Part model, mm, in its own coordinate system. Face numbers are marked on the shaded views. A direction names the side the tool comes from. Coordinates: 2 decimals unless noted, no trailing zeros. Write each loop counter-clockwise with the first axis right and the second up, starting at its lowest first coordinate (ties: lowest second). Pieces come first, ordered by that corner, then holes. Notation, with made-up numbers: M 41.25,52.25 L 69.25,52.25 A25 ccw 69.25,86.25 Z; hole C 84.25,-22.75 d10. An arc over 180 degrees is marked long. Use a Markdown table: item, result. Add a question column.
Q1. Wall check: L1, parallel to Z at x = 16.5, y = 18; L2, parallel to X at y = 5.5, z = 0; L3, parallel to Y at x = -3, z = 14. Give the ranges that are in metal, low to high. Write a range as from..to.
Q2. Slice it at A-A on x = -5. Write the cut outline in (y, z), then the cut area to 3 significant figures.
Q3. Pin check, flat tips, straight feed: pin 1 Ø3 at (x, z) = (4.5, 13.5) entering from -Y; pin 2 Ø6.5 at (x, y) = (-15, 19) entering from -Z; pin 3 Ø2.5 at (x, y) = (14.5, 20.5) entering from +Z. Stop position of each tip, or through.
Q4. Slice it at B-B on y = 6. Write the cut outline in (x, z), then the cut area to 3 significant figures.
Q5. Mould opens along Z. For the marked faces 1, 2 and 3 say: released by +Z, released by -Z, zero draft, split by the parting line, or undercut.
Q6. Slice it at C-C on x = 7. Write the cut outline in (y, z).
Q7. Slice it at D-D on z = 17.5. Write the cut outline in (x, y), then the cut area to 3 significant figures.
Q8. Tool access for the marked faces 4, 5 and 6: list every direction of +Z, -Z, +X, -X, +Y, -Y with a clear straight run to the whole face (end or side of a thin tool).
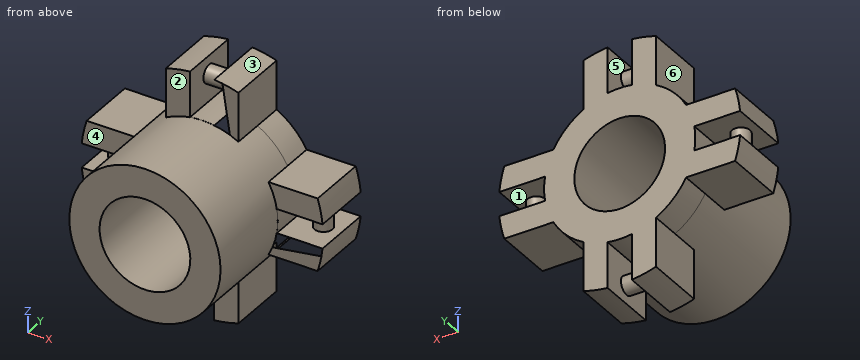
from build123d import *

# Parameters (mm, degrees)
SKETCH1_R           = 12.5
SKETCH1_R_2         = 7.5
BOSS_EXTRUDE1_DEPTH = 20
SKETCH2_R           = 7.5
BOSS_EXTRUDE2_DEPTH = 5
SKETCH3_R           = 1.5
BOSS_EXTRUDE3_DEPTH = 7
CIRPATTERN1_COUNT   = 4


with BuildPart() as part:
    # Sketch1 → Boss-Extrude1 (new body)
    with BuildSketch(Plane(origin=(0, 0, 0), x_dir=(1, 0, 0), z_dir=(0, 1, 0))):
        with Locations(Location((0, 0, 0), (0, 0, 270))):
            Circle(SKETCH1_R)
        with Locations(Location((0, 0, 0), (0, 0, 270))):
            Circle(SKETCH1_R_2, mode=Mode.SUBTRACT)
    extrude(amount=BOSS_EXTRUDE1_DEPTH)

    # Sketch2 → Boss-Extrude2 (add, symmetric)
    with BuildSketch(Plane(origin=(0, 20, 0), x_dir=(1, 0, 0), z_dir=(0, 1, 0))):
        with BuildLine():
            Line((-2, 19.899749), (-2, 12.338963))
            ThreePointArc((-2, 12.338963), (0, 12.5), (2, 12.338963))
            Line((2, 12.338963), (2, 19.899749))
            ThreePointArc((2, 19.899749), (4.021007, 19.591618), (6, 19.078784))
            Line((6, 19.078784), (6, 10.965856))
            ThreePointArc((6, 10.965856), (8.838835, 8.838835), (10.965856, 6))
            Line((10.965856, 6), (19.078784, 6))
            ThreePointArc((19.078784, 6), (19.591618, 4.021007), (19.899749, 2))
            Line((19.899749, 2), (12.338963, 2))
            ThreePointArc((12.338963, 2), (12.5, 0), (12.338963, -2))
            Line((12.338963, -2), (19.899749, -2))
            ThreePointArc((19.899749, -2), (19.591618, -4.021007), (19.078784, -6))
            Line((19.078784, -6), (10.965856, -6))
            ThreePointArc((10.965856, -6), (8.838835, -8.838835), (6, -10.965856))
            Line((6, -10.965856), (6, -19.078784))
            ThreePointArc((6, -19.078784), (4.021007, -19.591618), (2, -19.899749))
            Line((2, -19.899749), (2, -12.338963))
            ThreePointArc((2, -12.338963), (0, -12.5), (-2, -12.338963))
            Line((-2, -12.338963), (-2, -19.899749))
            ThreePointArc((-2, -19.899749), (-4.021007, -19.591618), (-6, -19.078784))
            Line((-6, -19.078784), (-6, -10.965856))
            ThreePointArc((-6, -10.965856), (-8.838835, -8.838835), (-10.965856, -6))
            Line((-10.965856, -6), (-19.078784, -6))
            ThreePointArc((-19.078784, -6), (-19.591618, -4.021007), (-19.899749, -2))
            Line((-19.899749, -2), (-12.338963, -2))
            ThreePointArc((-12.338963, -2), (-12.5, 0), (-12.338963, 2))
            Line((-12.338963, 2), (-19.899749, 2))
            ThreePointArc((-19.899749, 2), (-19.591618, 4.021007), (-19.078784, 6))
            Line((-19.078784, 6), (-10.965856, 6))
            ThreePointArc((-10.965856, 6), (-8.838835, 8.838835), (-6, 10.965856))
            Line((-6, 10.965856), (-6, 19.078784))
            ThreePointArc((-6, 19.078784), (-4.021007, 19.591618), (-2, 19.899749))
        make_face()
        with Locations(Location((0, 0, 0), (0, 0, 270))):
            Circle(SKETCH2_R, mode=Mode.SUBTRACT)
    extrude(amount=BOSS_EXTRUDE2_DEPTH, both=True)

    # Sketch3 → Boss-Extrude3 (add)
    with BuildSketch(Plane.XY.offset(-2)):
        with Locations(Location((-16.899749, 20, 0), (0, 0, 180))):
            Circle(SKETCH3_R)
    boss_extrude3 = extrude(amount=BOSS_EXTRUDE3_DEPTH)

    # CirPattern1: Boss-Extrude3 ×4 about axis
    cirpattern1_axis = Axis((0, 0, 0), (0, -1, 0))
    for i in range(1, CIRPATTERN1_COUNT):
        add(boss_extrude3.rotate(cirpattern1_axis, i * 360 / CIRPATTERN1_COUNT))


solid = part.part
Recorded:
| question | item | result |
|---|---|---|
| 1 | L1 | -6..-2, 2..6 |
| 1 | L2 | -12.5..-7.5, 7.5..12.5 |
| 1 | L3 | 15..25 |
| 2 | outline | M 0,-11.46 L 15,-11.46 L 15,-19.36 L 25,-19.36 L 25,-5.59 L 0,-5.59 Z; M 0,5.59 L 25,5.59 L 25,19.36 L 15,19.36 L 15,11.46 L 0,11.46 Z |
| 2 | area | 451 mm² |
| 3 | pin 1 | y = 15 |
| 3 | pin 2 | z = -6 |
| 3 | pin 3 | z = 6 |
| 4 | outline | C 0,0 d25; hole C 0,0 d15 |
| 4 | area | 314 mm² |
| 5 | face 1 | undercut |
| 5 | face 2 | zero draft |
| 5 | face 3 | released by +Z |
| 6 | outline | M 0,-10.36 L 25,-10.36 L 25,-2.69 L 0,-2.69 Z; M 0,2.69 L 25,2.69 L 25,10.36 L 0,10.36 Z |
| 7 | outline | M -6,15 L -2,15 L -2,18.63 L 2,18.63 L 2,15 L 6,15 L 6,25 L 2,25 L 2,21.37 L -2,21.37 L -2,25 L -6,25 Z |
| 7 | area | 91.0 mm² |
| 8 | face 4 | +Z, -X, -Y |
| 8 | face 5 | none |
| 8 | face 6 | +Z, -X, +Y, -Y |
